Work out the finished part from the listing and answer in its coordinate system (mm). Face numbers are marked on the shaded views. A direction names the side the tool comes from. Give positions to 0.01 mm unless a question says otherwise; leave off trailing zeros. Loops run counter-clockwise (first coordinate to the right, second up) from the corner with the lowest first, then second, coordinate; pieces in that order, holes last. Notation, with made-up numbers: M -8.75,-6 L -4.75,-6 A15 cw -4.75,14 Z; hole C 49.5,-1 d6. An arc over 180 degrees is marked long. Write item = value, one per line. Start each with the question number.
1. Section C-C on x = 0 is taken. Determine the outline of the cut face in (y, z) (3 decimals).
2. Section B-B on z = 6 is taken. Determine the outline of the cut face in (x, y), plus the area to 3 significant figures.
3. Flat-ended cylindrical pins translate along their axes: pin 1 Ø1 at (x, y) = (11.5, 1) entering from -Z; pin 2 Ø4.5 at (y, z) = (16, 1) entering from +X; pin 3 Ø3 at (x, z) = (9, -1.5) entering from -Y; pin 4 Ø8 at (y, z) = (9, -5) entering from -X. Find the tip coordinate at first contact, or state that the pin passes through.
4. Section A-A on x = 10 is taken. Determine the outline of the cut face in (y, z).
5. For the marked faces 5, 6, 7 and 8, determine the directions among +Z, -Z, +X, -X, +Y, -Y from which every point of the face is accessible in a straight line to the end or side of a thin tool.
6. The mould has two halves that part along Z. Classify the marked faces 1, 2, 3 and 4: released by +Z, released by -Z, zero draft, split by the parting line, or undercut.
7. Consider L1, parallel to X at y = 3.75, z = 0 (3 decimals); L2, parallel to Y at x = 5, z = 5.75; L3, parallel to X at y = 12, z = 3. Determine where each line is inside the solid, lowest interval first. Write a range as [from, to].
8. Section D-D on x = -3.75 is taken. Determine the outline of the cut face in (y, z).
```python
from build123d import *

# Parameters (mm, degrees)
SKETCH_2_W          = 5.9
SKETCH_2_H          = 15.7
EXTRUDE_1_DEPTH     = 33.5
SKETCH_3_R          = 0.975
CUT_EXTRUDE_1_DEPTH = 10
SKETCH_4_W          = 3.8
SKETCH_4_H          = 3.8
EXTRUDE_2_DEPTH     = 13
SKETCH_5_W          = 3.8
SKETCH_5_H          = 4
EXTRUDE_3_DEPTH     = 4
FILLET_1_R          = 0.8
FILLET_2_R          = 0.5


with BuildPart() as part:
    # ｽｹｯﾁ2 → ﾎﾞｽ - 押し出し1 (new body)
    with BuildSketch(Plane(origin=(0, 0, 0), x_dir=(1, 0, 0), z_dir=(0, 1, 0))):
        Rectangle(SKETCH_2_W, SKETCH_2_H)
    extrude(amount=EXTRUDE_1_DEPTH)

    # ｽｹｯﾁ3 → ｶｯﾄ - 押し出し1 (cut)
    with BuildSketch(Plane.XZ):
        with Locations(Location((0, 0, 0), (0, 0, 270))):
            Circle(SKETCH_3_R)
    extrude(amount=-CUT_EXTRUDE_1_DEPTH, mode=Mode.SUBTRACT)

    # ｽｹｯﾁ4 → ﾎﾞｽ - 押し出し2 (add)
    with BuildSketch(Plane(origin=(2.95, 0, 0), x_dir=(0, 0, -1), z_dir=(1, 0, 0))):
        with Locations((-5.85, 1.9)):
            Rectangle(SKETCH_4_W, SKETCH_4_H)
        with Locations((5.85, 1.9)):
            Rectangle(SKETCH_4_W, SKETCH_4_H)
    extrude(amount=EXTRUDE_2_DEPTH)

    # ｽｹｯﾁ5 → ﾎﾞｽ - 押し出し3 (add)
    with BuildSketch(Plane.ZY.offset(2.95)):
        with Locations((-5.95, 2)):
            Rectangle(SKETCH_5_W, SKETCH_5_H)
        with Locations((5.95, 2)):
            Rectangle(SKETCH_5_W, SKETCH_5_H)
    extrude(amount=EXTRUDE_3_DEPTH)

    # ﾌｨﾚｯﾄ1
    fillet_1_edges = [part.edges().sort_by_distance(p)[0] for p in [
        (-4.95, 4, -4.05),
        (-4.95, 4, 4.05),
    ]]
    fillet(fillet_1_edges, radius=FILLET_1_R)

    # ﾌｨﾚｯﾄ2
    fillet_2_edges = [part.edges().sort_by_distance(p)[0] for p in [
        (9.45, 3.8, 7.75),
        (9.45, 3.8, 3.95),
        (9.45, 3.8, -3.95),
        (9.45, 3.8, -7.75),
    ]]
    fillet(fillet_2_edges, radius=FILLET_2_R)


solid = part.part
```
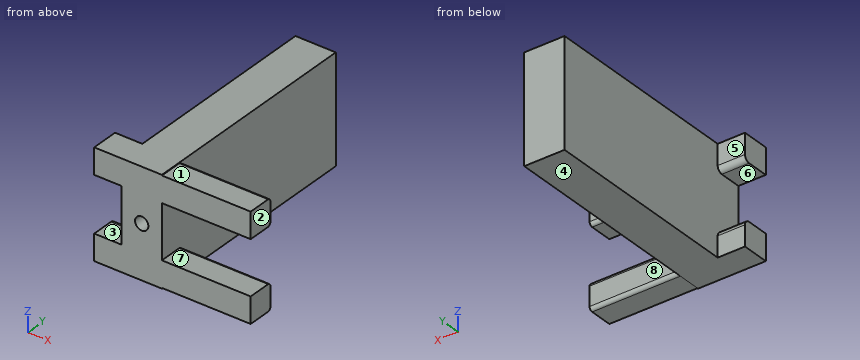
Verdict:
q1.outline = M 0,-7.85 L 33.5,-7.85 L 33.5,7.85 L 0,7.85 L 0,0.975 L 10,0.975 L 10,-0.975 L 0,-0.975 Z
q2.outline = M -6.95,0 L 15.95,0 L 15.95,3.8 L 2.95,3.8 L 2.95,33.5 L -2.95,33.5 L -2.95,4 L -6.95,4 Z
q2.area = 263 mm2
q3.pin_1 = -7.75
q3.pin_2 = 2.95
q3.pin_3 = through
q3.pin_4 = -2.95
q4.outline = M 0,-7.75 L 3.3,-7.75 A0.5 ccw 3.8,-7.25 L 3.8,-4.45 A0.5 ccw 3.3,-3.95 L 0,-3.95 Z; M 0,3.95 L 3.3,3.95 A0.5 ccw 3.8,4.45 L 3.8,7.25 A0.5 ccw 3.3,7.75 L 0,7.75 Z
q5.face_5 = +Z, -Z, -X, +Y
q5.face_6 = -X, +Y, -Y
q5.face_7 = +X, +Y, -Y
q5.face_8 = +Z, -Z, +X, +Y
q6.face_1 = released by +Z
q6.face_2 = zero draft
q6.face_3 = undercut
q6.face_4 = released by -Z
q7.L1 = [-2.95, -0.975], [0.975, 2.95]
q7.L2 = [0, 3.8]
q7.L3 = [-2.95, 2.95]
q8.outline = M 0,-7.85 L 4,-7.85 L 4,-4.85 A0.8 ccw 3.2,-4.05 L 0,-4.05 Z; M 0,4.05 L 3.2,4.05 A0.8 ccw 4,4.85 L 4,7.85 L 0,7.85 Z
